Source: three-view drawing plus pictorial views. Frame: mm from the lowest corner of the part. A direction names the side the tool comes from. Round coordinates to 2 decimals unless told otherwise and drop trailing zeros. Loops run counter-clockwise (first coordinate to the right, second up) from the corner with the lowest first, then second, coordinate; pieces in that order, holes last. Notation, with made-up numbers: (-27.75, 23.5) -> (19.25, 23.5) arc R19 ccw to (19.25, 42.5) -> close; hole circle Ø4 at (12.5, 88.25). An arc over 180 degrees is marked (long way). One line per question, with ' | ' between items. Start each with the question number.
Q1. Material intervals for L1, parallel to X at y = 0.05, z = 5; L2, parallel to X at y = 1.4, z = 5; L3, parallel to Z at x = 5.75, y = 1.35, sorted ascending.
Q2. Cut plane A-A on y = 0.9. Return loops of the section in (x, z).
Q3. Cut plane B-B on z = 8.5. Return loops of the section in (x, y), and give its area (3 significant figures).
Q4. Access query for the marked faces 3 and 4. Directions: +Z, -Z, +X, -X, +Y, -Y. A direction counts if a zero-diameter tool reaches every point of the face in a straight line with its end or side. Return the directions, or none.
Q5. Mould query, pull axis X, two halves, no side actions, for the marked faces 1 and 2. Classes: pulls with the +X half, pulls with the -X half, needs draft (parallel to the pull), parting line crosses it, or undercut.
Q6. Contact query for a flat-ended pin moving along its axis: P1, Ø1, axis at x = 6, y = 3.5, coming from the -Z side. Output: stop coordinate, or through.
Q7. Cut plane C-C on x = 1.5. Return loops of the section in (y, z).
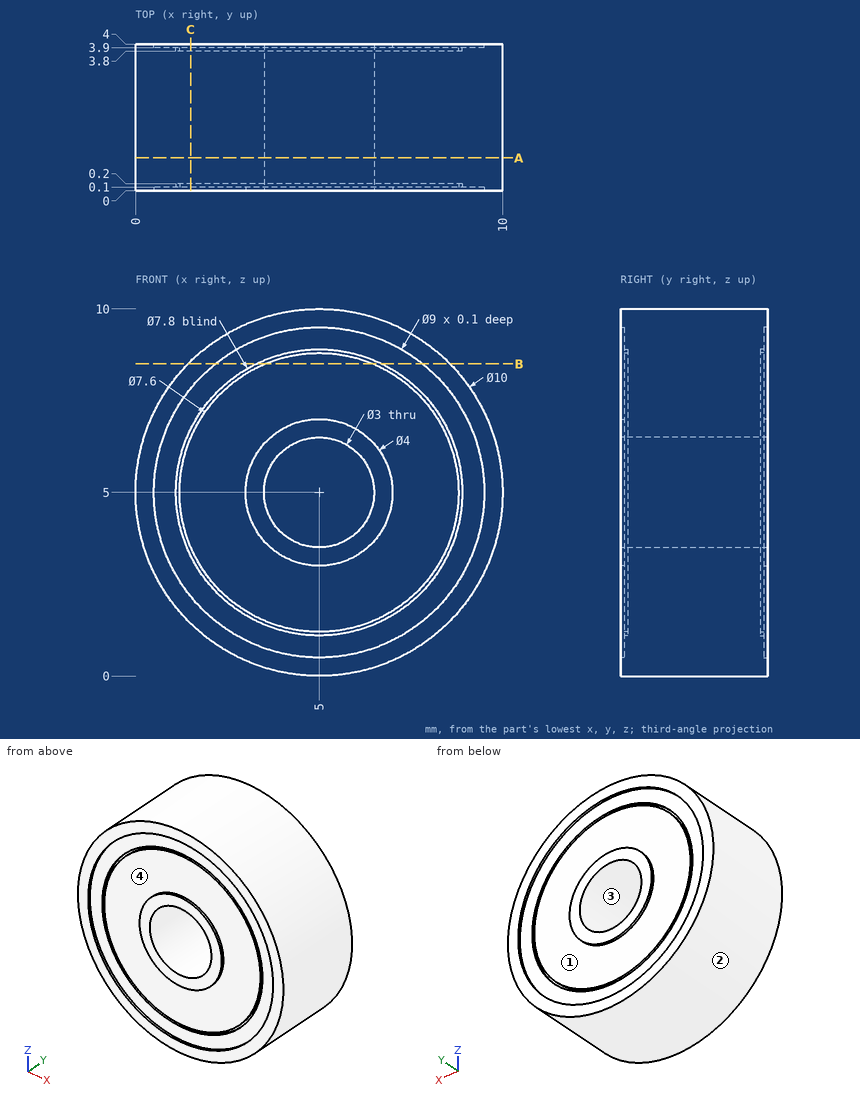
Results:
1) L1: 0 to 0.5, 3 to 3.5, 6.5 to 7, 9.5 to 10 | L2: 0 to 3.5, 6.5 to 10 | L3: 0.06 to 3.7, 6.3 to 9.94
2) outline: circle Ø10 at (5, 5); hole circle Ø3 at (5, 5)
3) outline: (1.43, 0) -> (2.17, 0) -> (2.17, 0.1) -> (3.28, 0.1) -> (3.28, 0.2) -> (3.52, 0.2) -> (3.52, 0.1) -> (6.48, 0.1) -> (6.48, 0.2) -> (6.72, 0.2) -> (6.72, 0.1) -> (7.83, 0.1) -> (7.83, 0) -> (8.57, 0) -> (8.57, 4) -> (7.83, 4) -> (7.83, 3.9) -> (6.72, 3.9) -> (6.72, 3.8) -> (6.48, 3.8) -> (6.48, 3.9) -> (3.52, 3.9) -> (3.52, 3.8) -> (3.28, 3.8) -> (3.28, 3.9) -> (2.17, 3.9) -> (2.17, 4) -> (1.43, 4) -> close | area: 27.3 mm^2
4) face 3: +Y, -Y | face 4: -Y
5) face 1: undercut | face 2: parting line crosses it
6) P1: z = 0.03
7) outline: (0, 1.43) -> (4, 1.43) -> (4, 2.17) -> (3.9, 2.17) -> (3.9, 3.28) -> (3.8, 3.28) -> (3.8, 3.52) -> (3.9, 3.52) -> (3.9, 6.48) -> (3.8, 6.48) -> (3.8, 6.72) -> (3.9, 6.72) -> (3.9, 7.83) -> (4, 7.83) -> (4, 8.57) -> (0, 8.57) -> (0, 7.83) -> (0.1, 7.83) -> (0.1, 6.72) -> (0.2, 6.72) -> (0.2, 6.48) -> (0.1, 6.48) -> (0.1, 3.52) -> (0.2, 3.52) -> (0.2, 3.28) -> (0.1, 3.28) -> (0.1, 2.17) -> (0, 2.17) -> close
